Geometry: final body of the model. Coordinates: model frame, mm. Face numbers are marked on the shaded views. A direction names the side the tool comes from. Round coordinates to 2 decimals unless told otherwise and drop trailing zeros. Loops run counter-clockwise (first coordinate to the right, second up) from the corner with the lowest first, then second, coordinate; pieces in that order, holes last. Notation, with made-up numbers: (-18, -23) - (22, -23) arc R26 ccw to (22, -3) - close; hole circle Ø9 at (52.5, 81). An arc over 180 degrees is marked (long way). Answer as a JSON object with one key per item and string values. Group by question number.
Item 1: Section B-B (x = 19). Return the cut outline in (y, z), plus the area to 3 significant figures.
Item 2: Section A-A (y = -42.5). Return the cut outline in (x, z), plus the area to 3 significant figures.
Item 3: Draft query along Z for the marked faces 1, 2 and 3. Return one class per face: released by +Z, released by -Z, zero draft, split by the parting line, or undercut.
Item 4: Section C-C (z = -12). Return the cut outline in (x, y).
Item 5: Reachability of the marked faces 4 and 5 from +Z, -Z, +X, -X, +Y, -Y: full face, straight path, thin tool, end or side. Return the list, or none.
Item 6: Line query: line 1 (X direction, y = -52.5, z = 18.5); line 2 (Z direction, x = 41.5, y = -13.5); line 3 (Y direction, x = -57.5, z = -5). Output: solid intervals per line, ascending.
Item 7: Section D-D (z = 0). Return the cut outline in (x, y), plus the area to 3 significant figures.
Item 8: First-contact query: pin 1 (3 mm diameter, centred on x = 2, z = 33.5, fed in from -Y); pin 2 (15.5 mm diameter, centred on y = -31.54, z = 0, fed in from +X) (3 decimals). Flat tips, straight axial feed; report the tip coordinate or a pass-through.
```python
from build123d import *

# Parameters (mm, degrees)
F0_W     = 133.384466
F0_H     = 87.411344
F1_DEPTH = 63.5
F4_W     = 110.828802
F4_H     = 67.344964
F5_DEPTH = 63.501
F6_W     = 55.005372
F6_H     = 22.744318
F2_DEPTH = 87.412344
F3_R     = 8.477147
F7_DEPTH = 133.385466


with BuildPart() as f1:
    # F0 (on Front) → F1 (new body)
    with BuildSketch(Plane.XZ):
        Rectangle(F0_W, F0_H)
    extrude(amount=F1_DEPTH)

    # F4 (on face) → F5 (cut, through all)
    with BuildSketch(Plane.XZ.offset(63.5)):
        Rectangle(F4_W, F4_H)
    extrude(amount=-F5_DEPTH, mode=Mode.SUBTRACT)

    # F6 (on face) → F2 (cut, through all)
    with BuildSketch(Plane(origin=(0, 0, -43.705672), x_dir=(1, 0, 0), z_dir=(0, 0, -1))):
        with Locations((0, 74.872159)):
            Rectangle(F6_W, F6_H)
        with Locations((0, 52.127841)):
            Rectangle(F6_W, F6_H)
    extrude(amount=-F2_DEPTH, mode=Mode.SUBTRACT)

    # F3 (on face) → F7 (cut, through all)
    with BuildSketch(Plane.YZ.offset(66.692233)):
        with Locations((-31.544417, 0)):
            Circle(F3_R)
    extrude(amount=-F7_DEPTH, mode=Mode.SUBTRACT)


solid = f1.part
```
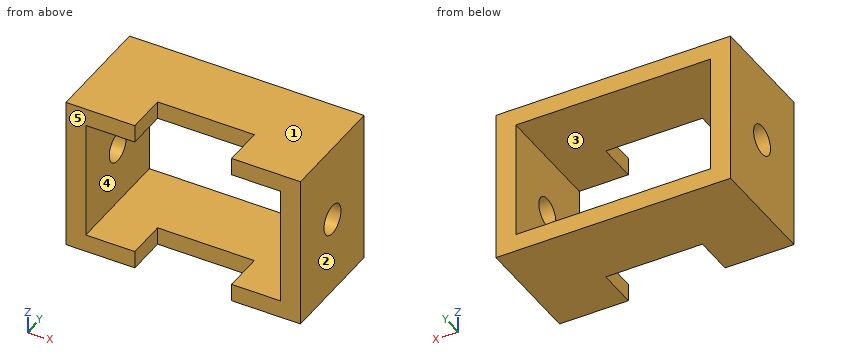
Values:
{
 "1": {"outline": "(-40.76, -43.71) - (0, -43.71) - (0, -33.67) - (-40.76, -33.67) - close; (-40.76, 33.67) - (0, 33.67) - (0, 43.71) - (-40.76, 43.71) - close", "area": "818 mm^2"},
 "2": {"outline": "(-66.69, -43.71) - (-27.5, -43.71) - (-27.5, -33.67) - (-55.41, -33.67) - (-55.41, 33.67) - (-27.5, 33.67) - (-27.5, 43.71) - (-66.69, 43.71) - close; (27.5, -43.71) - (66.69, -43.71) - (66.69, 43.71) - (27.5, 43.71) - (27.5, 33.67) - (55.41, 33.67) - (55.41, -33.67) - (27.5, -33.67) - close", "area": "3,090 mm^2"},
 "3": {"face 1": "released by +Z", "face 2": "zero draft", "face 3": "undercut"},
 "4": {"outline": "(-66.69, -63.5) - (-55.41, -63.5) - (-55.41, 0) - (-66.69, 0) - close; (55.41, -63.5) - (66.69, -63.5) - (66.69, 0) - (55.41, 0) - close"},
 "5": {"face 4": "+Y, -Y", "face 5": "+Z, -Z, +X, -X, -Y"},
 "6": {"line 1": "x = -66.69 to -55.41, 55.41 to 66.69", "line 2": "z = -43.71 to -33.67, 33.67 to 43.71", "line 3": "y = -63.5 to -38.39, -24.7 to 0"},
 "7": {"outline": "(-66.69, -63.5) - (-55.41, -63.5) - (-55.41, -40.02) - (-66.69, -40.02) - close; (-66.69, -23.07) - (-55.41, -23.07) - (-55.41, 0) - (-66.69, 0) - close; (55.41, -63.5) - (66.69, -63.5) - (66.69, -40.02) - (55.41, -40.02) - close; (55.41, -23.07) - (66.69, -23.07) - (66.69, 0) - (55.41, 0) - close", "area": "1,050 mm^2"},
 "8": {"pin 1": "stops at y = -40.76", "pin 2": "passes through"}
}
